Model file for the job. Use its own axes, mm. A direction names the side the tool comes from. Round coordinates to 2 decimals unless told otherwise and drop trailing zeros. Order: outer loops, then holes, each group sorted by start corner. A loop starts at its lowest first (then second) coordinate and runs counter-clockwise, first axis right, second up. Notation, with made-up numbers: (49.25, -37) - (104.25, -37) arc R30 ccw to (104.25, -1) - close; hole circle Ø1 at (37.5, 29.5). An arc over 180 degrees is marked (long way). Answer as CSV lines item,"result". Start each with the question number.
1. Band-saw the part on C-C on z = -98. List the corners of the cut face in (x, y).
2. Wall check: line 1 along X through (y, z) = (35.5, -75.5); line 2 along Z through (x, y) = (8, 26); line 3 along Y through (x, z) = (67, -116.5). Give the ranges that are in metal, low to high. Write a range as [from, to].
3. Pin check, flat tips, straight feed: pin 1 Ø8 at (x, y) = (80, 78) entering from -Z; pin 2 Ø11 at (x, z) = (14.5, -185.5) entering from +Y; pin 3 Ø4.5 at (x, z) = (66, -59.5) entering from -Y; pin 4 Ø1.5 at (x, y) = (37.5, 21.5) entering from +Z. Stop position of each tip, or through.
4. Band-saw the part on D-D on y = 28. List the corners of the cut face in (x, z).
5. Band-saw the part on A-A on y = 47. List the corners of the cut face in (x, z), then the cut area to 3 significant figures.
6. 3-axis set-ups, long thin cutter, end or side, ignore diameter. For faces 1 (the face through (50, 42, -99)), 2 (the face through (51, 54, -50)), 3 (the face through (68, 20, -74)), 4 (the face through (81, 22, -99)), 5 (the face through (51, 50, -6)): which of +Z, -Z, +X, -X, +Y, -Y reach the whole face in a straight line?
7. Pull direction Z, two halves, no side cores. Call faces 6 (the face through (19, 22, -99)), 7 (the face through (25, 10, -74)), 8 (the face through (50.7, 76.81, -23.78)): released by +Z, released by -Z, zero draft, split by the parting line, or undercut.
8. Band-saw the part on B-B on x = 92. List the corners of the cut face in (y, z).
Autodesk Fusion 360 part; units mm, degrees
sketch "Sketch1" plane through (0, 0, 0) normal (0, 0, 1) x (1, 0, 0)
  line L0 (0, 0) -> (100, 0)
  line L1 (100, 0) -> (100, 50)
  line L2 (100, 50) -> (0, 50)
  line L3 (0, 50) -> (0, 0)
  line L4 (0, 0) -> (25, 0)
  line L5 (25, 0) -> (25, 20)
  line L6 (25, 20) -> (40, 20)
  line L7 (40, 20) -> (40, 40)
  line L8 (40, 40) -> (50, 40)
  line L9 (0, 50) -> (100, 50)
  line L10 (75, 20) -> (60, 20)
  line L11 (60, 20) -> (60, 40)
  line L12 (60, 40) -> (50, 40)
  line L13 (75, 0) -> (75, 20)
  dimension "d1" = 100
  dimension "d2" = 50
  dimension "d3" = 25
  dimension "d4" = 20
  dimension "d5" = 90
  dimension "d6" = 15
  dimension "d7" = 20
extrude "Extrude1" add sketch "Sketch1" against normal blind 50 contours L0 L1 L2 L3 L4 L5 L6 L7 L8 L9 L10 L11 L12 L13
sketch "Sketch2" plane through (0, 0, -50) normal (0, 0, -1) x (-1, 0, 0)
  line L0 (-100, 50) -> (-100, 0)
  line L1 (-100, 0) -> (-75, 0)
  line L2 (-75, 0) -> (-75, 20)
  line L3 (-75, 20) -> (-60, 20)
  line L4 (-60, 20) -> (-60, 40)
  line L5 (-60, 40) -> (-40, 40)
  line L6 (-40, 40) -> (-40, 20)
  line L7 (-40, 20) -> (-25, 20)
  line L8 (-25, 20) -> (-25, 0)
  line L9 (-25, 0) -> (0, 0)
  line L10 (0, 0) -> (0, 50)
  line L11 (0, 50) -> (-100, 50)
  line L12 (-75, 20) -> (-25, 20)
  line L13 (0, 0) -> (-100, 0)
  line L14 (-100, 20) -> (-100, 0)
  line L15 (0, 20) -> (0, 0)
  line L16 (-100, 20) -> (-100, 22)
  line L17 (-100, 22) -> (-62, 22)
  line L18 (-62, 40) -> (-62, 22)
  line L19 (-62, 40) -> (-62, 42)
  line L20 (-62, 42) -> (-40, 42)
  line L21 (-50, 20) -> (-50, 22)
  line L22 (-38, 40) -> (-38, 22)
  line L23 (-38, 42) -> (-60, 42)
  line L24 (-38, 40) -> (-38, 42)
  line L25 (0, 22) -> (-38, 22)
  dimension "d10" = 2
  dimension "d11" = 2
  dimension "d12" = 2
extrude "Extrude2" add sketch "Sketch2" along normal blind 100 contours L0 L1 L2 L3 L4 L5 L6 L7 L8 L9 L10 L12 L13 L14 L15 L16 L17 L18 L19 L20 L22 L23 L24 L25
sketch "Sketch3" plane through (0, 0, -150) normal (0, 0, -1) x (-1, 0, 0)
  line L0 (0, 0) -> (0, 22)
  line L1 (0, 22) -> (-38, 22)
  line L2 (-38, 22) -> (-38, 42)
  line L3 (-38, 42) -> (-62, 42)
  line L4 (-62, 42) -> (-62, 22)
  line L5 (-62, 22) -> (-100, 22)
  line L6 (-100, 22) -> (-100, 0)
  line L7 (-100, 0) -> (-75, 0)
  line L8 (-75, 0) -> (-75, 20)
  line L9 (-75, 20) -> (-60, 20)
  line L10 (-60, 20) -> (-60, 40)
  line L11 (-60, 40) -> (-40, 40)
  line L12 (-40, 40) -> (-40, 20)
  line L13 (-40, 20) -> (-25, 20)
  line L14 (-25, 20) -> (-25, 0)
  line L15 (-25, 0) -> (0, 0)
  line L16 (-100, 0) -> (0, 0)
  line L17 (0, 0) -> (0, 60)
  line L18 (-100, 60) -> (-100, 0)
  arc A0 (-22.5, 60) -> (-77.5, 60) centre (-50, 60) ccw
  line L19 (0, 60) -> (-22.5, 60)
  line L20 (-77.5, 60) -> (-100, 60)
  dimension "d15" = 60
extrude "Extrude3" add sketch "Sketch3" along normal blind 50
sketch "Sketch4" plane through (100, 0, 0) normal (1, 0, 0) x (0, 0, -1)
  line L0 (0, 50) -> (0, 0)
  line L1 (0, 0) -> (200, 0)
  line L2 (200, 0) -> (200, 60)
  line L3 (200, 60) -> (150, 60)
  line L4 (150, 60) -> (150, 22)
  line L5 (150, 22) -> (50, 22)
  line L6 (50, 22) -> (50, 50)
  line L7 (50, 50) -> (0, 50)
  line L8 (50, 50) -> (50, 87.5)
  line L9 (12.5, 50) -> (50, 50)
  arc A0 (50, 87.5) -> (12.5, 50) centre (50, 50) ccw
  dimension "d19" = 75
extrude "Extrude4" add sketch "Sketch4" against normal blind 100 contours L7 L8 L9 A0
Reply:
1,outline,"(0, 0) - (25, 0) - (25, 20) - (40, 20) - (40, 40) - (60, 40) - (60, 20) - (75, 20) - (75, 0) - (100, 0) - (100, 22) - (62, 22) - (62, 42) - (38, 42) - (38, 22) - (0, 22) - close"
2,line 1,"x = [38, 40], [60, 62]"
2,line 2,"z = [-200, -150], [-50, 0]"
2,line 3,"y = [20, 22]"
3,pin 1,"stops at z = -50"
3,pin 2,"stops at y = 60"
3,pin 3,"stops at y = 20"
3,pin 4,"stops at z = 0"
4,outline,"(0, -200) - (100, -200) - (100, -150) - (62, -150) - (62, -50) - (100, -50) - (100, 0) - (60, 0) - (60, -150) - (40, -150) - (40, 0) - (0, 0) - (0, -50) - (38, -50) - (38, -150) - (0, -150) - close"
5,outline,"(0, -200) - (100, -200) - (100, -150) - (0, -150) - close; (0, -50) - (100, -50) - (100, 0) - (0, 0) - close"
5,area,"10,000 mm2"
6,face 1,"+X, -X, +Y"
6,face 2,"+Y"
6,face 3,"+Z, -Y"
6,face 4,"+X, +Y"
6,face 5,"+Z, +X, -X, +Y"
7,face 6,"undercut"
7,face 7,"zero draft"
7,face 8,"released by +Z"
8,outline,"(0, -200) - (60, -200) - (60, -150) - (22, -150) - (22, -50) - (87.5, -50) arc R37.5 ccw to (50, -12.5) - (50, 0) - (0, 0) - close"
